Autodesk Inventor part; units mm, degrees
ref_plane "YZ Plane" through (0, 0, 0) normal (1, 0, 0) x (0, 1, 0)
ref_plane "XZ Plane" through (0, 0, 0) normal (0, 1, 0) x (-1, 0, 0)
ref_plane "XY Plane" through (0, 0, 0) normal (0, 0, 1) x (1, 0, 0)
sketch "草圖1" plane through (0, 0, 0) normal (0, 1, 0) x (-1, 0, 0)
  line L0 (0, -10) -> (-20, -10)
  line L1 (-20, -10) -> (-20, 0)
  line L2 (-20, 0) -> (-30, 0)
  line L3 (-30, 0) -> (-60, -40)
  line L4 (-60, -40) -> (0, -40)
  line L5 (0, -40) -> (0, -10)
  point P0 (0, 0)
  dimension "d0" = 10
  dimension "d1" = 20
  dimension "d2" = 10
  dimension "d3" = 0
  dimension "d4" = 10
  dimension "d5" = 30
  dimension "d6" = 60
extrude "擠出1" add sketch "草圖1" along normal blind 10
sketch "草圖2" plane through (0, 0, -40) normal (-1, 0, 0) x (0, 0, 1)
  line L0 (40, 10) -> (0, 10)
  line L1 (0, 10) -> (0, 30)
  line L2 (0, 30) -> (20, 20)
  line L3 (20, 20) -> (20, 10)
  line L4 (20, 10) -> (0, 10)
  point P0 (40, 0)
  dimension "d9" = 20
  dimension "d10" = 20
  dimension "d11" = 10
extrude "擠出2" add sketch "草圖2" against normal blind 20
properties part number "43 (22000.000 mm^3)"
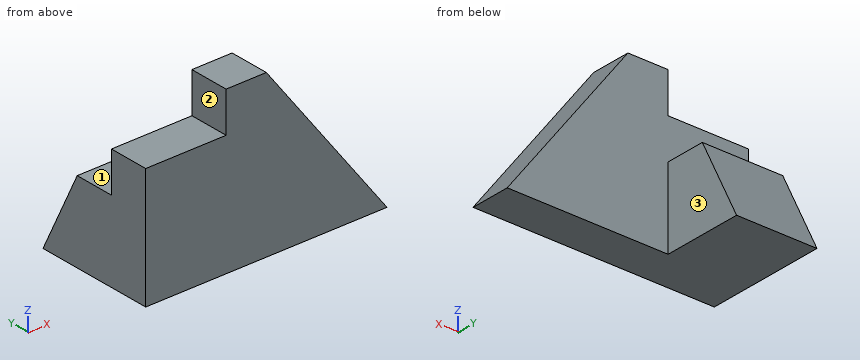
The model under review builds one solid part; all positions refer to its coordinate system, in mm. Face numbers are marked on the shaded views. A direction names the side the tool comes from. Give positions to 0.01 mm unless a question says otherwise; leave off trailing zeros. Order: outer loops, then holes, each group sorted by start corner. A loop starts at its lowest first (then second) coordinate and runs counter-clockwise, first axis right, second up. Notation, with made-up numbers: M 8,-22 L 12,-22 A18 ccw 12,2 Z; hole C 85.25,67 d1. An arc over 180 degrees is marked long. Use one line per item in the form item = value. Start each with the question number.
Item 1: We need section A-A on z = -29. Give the boundary of the cut face in (x, y).
Item 2: Insertion check: pin 1 Ø1 at (x, y) = (13, 26.5) entering from +Z; pin 2 Ø5 at (x, y) = (6, 4) entering from +Z; pin 3 Ø1 at (x, z) = (19, -7.5) entering from -Y; pin 4 Ø12 at (x, z) = (30, -28) entering from +Y. Each pin has a flat end and moves straight along its axis. Give the tip position at first contact, or say it passes through.
Item 3: For the marked faces 1, 2 and 3, list the 3-axis set-ups (+Z, -Z, +X, -X, +Y, -Y) from which the entire face can be reached by the end or side of a thin tool; tool diameter is ignored.
Item 4: We need section B-B on y = 8.25. Give the boundary of the cut face in (x, z).
Item 5: We need section C-C on x = 55. Give the boundary of the cut face in (y, z), plus the area to 3 significant figures.
Item 6: We need section D-D on y = 19. Give the boundary of the cut face in (x, z), plus the area to 3 significant figures.
Item 7: To check wall thickness, follow line 1 along X through (y, z) = (24.25, -33.5); line 2 along Y through (x, z) = (42, -36); line 3 along Z through (x, y) = (13.5, 2.5). State the ranges of each line that lie inside material, in increasing order. Write a range as from..to.
Completed:
q1.outline = M 0,0 L 51.75,0 L 51.75,10 L 20,10 L 20,24.5 L 0,24.5 Z
q2.pin_1 = -32
q2.pin_2 = -10
q2.pin_3 = through
q2.pin_4 = 10
q3.face_1 = +Z, +X, -X, +Y
q3.face_2 = +Z, -X, +Y, -Y
q3.face_3 = +Z, -Z, +X, +Y
q4.outline = M 0,-40 L 60,-40 L 30,0 L 20,0 L 20,-10 L 0,-10 Z
q5.outline = M 0,-40 L 10,-40 L 10,-33.33 L 0,-33.33 Z
q5.area = 66.7 mm²
q6.outline = M 0,-40 L 20,-40 L 20,-20 L 0,-20 Z
q6.area = 400 mm²
q7.line_1 = 0..20
q7.line_2 = 0..10
q7.line_3 = -40..-10
